Answer from the drawing. Dimensions are ordinates in mm from the lowest x, y and z of the part. A direction names the side the tool comes from. Coordinates: 2 decimals unless noted, no trailing zeros. Write each loop counter-clockwise with the first axis right and the second up, starting at its lowest first coordinate (ties: lowest second). Pieces come first, ordered by that corner, then holes.
(1) Find the intervals of material crossed by probe 1 along Y at (x, z) = (15, 2.6); probe 2 along Y at (x, z) = (42, 0.7); probe 3 along X at (y, z) = (20.5, 4.3), in increasing order.
(2) Section C-C on z = 2.55 is taken. Write down the section's boundary in (x, y).
(3) Which of the six approach directions +Z, -Z, +X, -X, +Y, -Y give full straight-line access (tool end or side, diameter ignored) to the marked faces 1 and 2?
(4) Section A-A on y = 53.5 is taken. Write down the section's boundary in (x, z).
(5) Section D-D on x = 42 is taken. Write down the section's boundary in (y, z).
(6) Section B-B on x = 15 is taken. Write down the section's boundary in (y, z).
(7) Given pin 1 (1.3 mm diameter, centred on x = 3.5, z = 1.5, fed in from -Y); pin 2 (1.3 mm diameter, centred on y = 3, z = 2, fed in from +X), each flat-ended and moving along its own axis, determine where each tip first touches the part or whether it passes through.
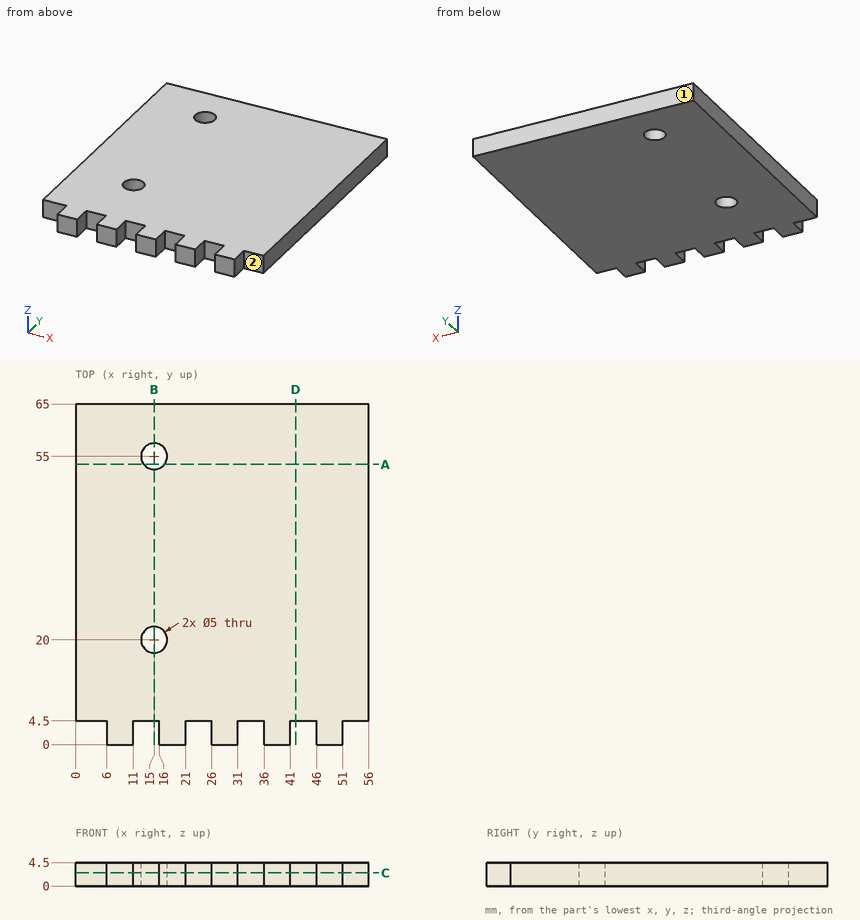
Response:
1. probe 1: y = 4.5 to 17.5, 22.5 to 52.5, 57.5 to 65
1. probe 2: y = 4.5 to 65
1. probe 3: x = 0 to 12.55, 17.45 to 56
2. outline: (0, 4.5) - (6, 4.5) - (6, 0) - (11, 0) - (11, 4.5) - (16, 4.5) - (16, 0) - (21, 0) - (21, 4.5) - (26, 4.5) - (26, 0) - (31, 0) - (31, 4.5) - (36, 4.5) - (36, 0) - (41, 0) - (41, 4.5) - (46, 4.5) - (46, 0) - (51, 0) - (51, 4.5) - (56, 4.5) - (56, 65) - (0, 65) - close; hole circle Ø5 at (15, 20); hole circle Ø5 at (15, 55)
3. face 1: +Z, -Z, +X, -X, +Y
3. face 2: +Z, -Z, +X, -Y
4. outline: (0, 0) - (13, 0) - (13, 4.5) - (0, 4.5) - close; (17, 0) - (56, 0) - (56, 4.5) - (17, 4.5) - close
5. outline: (4.5, 0) - (65, 0) - (65, 4.5) - (4.5, 4.5) - close
6. outline: (4.5, 0) - (17.5, 0) - (17.5, 4.5) - (4.5, 4.5) - close; (22.5, 0) - (52.5, 0) - (52.5, 4.5) - (22.5, 4.5) - close; (57.5, 0) - (65, 0) - (65, 4.5) - (57.5, 4.5) - close
7. pin 1: stops at y = 4.5
7. pin 2: stops at x = 51
